The model under review builds one solid part; all positions refer to its coordinate system, in mm. Coordinates: 2 decimals unless noted, no trailing zeros. Order: outer loops, then holes, each group sorted by start corner. A loop starts at its lowest first (then second) coordinate and runs counter-clockwise, first axis right, second up. Notation, with made-up numbers: (-11.5, 41.5) -> (23.5, 41.5) arc R17 ccw to (23.5, 56.5) -> close; hole circle Ø6 at (82.25, 17). An arc over 180 degrees is marked (long way). Put each result on its own line as item: value.
from build123d import *

# Parameters (mm, degrees)
ESQUISSE1_R             = 32.5
BOSS_EXTRU_2_DEPTH      = 5
ESQUISSE2_R             = 2
ENL_V_MAT_EXTRU_1_DEPTH = 5
ENL_V_MAT_EXTRU_2_DEPTH = 10


with BuildPart() as part:
    # Esquisse1 → Boss.-Extru.2 (new body)
    with BuildSketch(Plane.XY):
        with BuildLine():
            Line((-2, 166.988023523), (-2, 99.979998))
            ThreePointArc((-2, 99.979998), (100, 0), (-2, -99.979998))
            Line((-2, -99.979998), (-2, -166.988023523))
            ThreePointArc((-2, -166.988023523), (167, 0), (-2, 166.988023523))
        make_face()
        with Locations((33.922197974, 129.118296475)):
            Circle(ESQUISSE1_R, mode=Mode.SUBTRACT)
        with Locations((93.936633435, 94.858625854)):
            Circle(ESQUISSE1_R, mode=Mode.SUBTRACT)
        with Locations((128.780823828, 35.18166304)):
            Circle(ESQUISSE1_R, mode=Mode.SUBTRACT)
        with Locations((129.118296475, -33.922197974)):
            Circle(ESQUISSE1_R, mode=Mode.SUBTRACT)
        with Locations((94.858625854, -93.936633435)):
            Circle(ESQUISSE1_R, mode=Mode.SUBTRACT)
        with Locations((35.18166304, -128.780823828)):
            Circle(ESQUISSE1_R, mode=Mode.SUBTRACT)
    extrude(amount=BOSS_EXTRU_2_DEPTH)

    # Esquisse2 → Enlèv. mat.-Extru.1 (cut)
    with BuildSketch(Plane(origin=(0, 0, 0), x_dir=(-1, 0, 0), z_dir=(0, 0, -1))):
        with Locations((-77.031940381, 134.503086066)):
            Circle(ESQUISSE2_R)
        with Locations((-54.667828657, 95.453803014)):
            Circle(ESQUISSE2_R)
        with Locations((-77.96711923, -133.963160305)):
            Circle(ESQUISSE2_R)
        with Locations((-55.33150397, -95.070629894)):
            Circle(ESQUISSE2_R)
        with Locations((-134.503086066, -77.031940381)):
            Circle(ESQUISSE2_R)
        with Locations((-95.453803014, -54.667828657)):
            Circle(ESQUISSE2_R)
        with Locations((-154.999059611, 0.53992576)):
            Circle(ESQUISSE2_R)
        with Locations((-109.999332627, 0.38317312)):
            Circle(ESQUISSE2_R)
        with Locations((-133.963160305, 77.96711923)):
            Circle(ESQUISSE2_R)
        with Locations((-95.070629894, 55.33150397)):
            Circle(ESQUISSE2_R)
    extrude(amount=-ENL_V_MAT_EXTRU_1_DEPTH, mode=Mode.SUBTRACT)

    # Esquisse3 → Enlèv. mat.-Extru.2 (cut)
    with BuildSketch(Plane.XY.offset(5)):
        Polygon((0, 0), (77.031940381, 134.503086066), (82.995703507, 144.916228213), (91.624548615, 157.474747761), (25.313830581, 172.484842021), (-36.151543954, 181.613524578), (-51.569744744, -183.237067308), (77.031940381, -179.146608877), (82.995703507, -170.83045621), (84.003283299, -144.334501748), (77.96711923, -133.963160305), align=None)
    extrude(amount=-ENL_V_MAT_EXTRU_2_DEPTH, mode=Mode.SUBTRACT)


solid = part.part
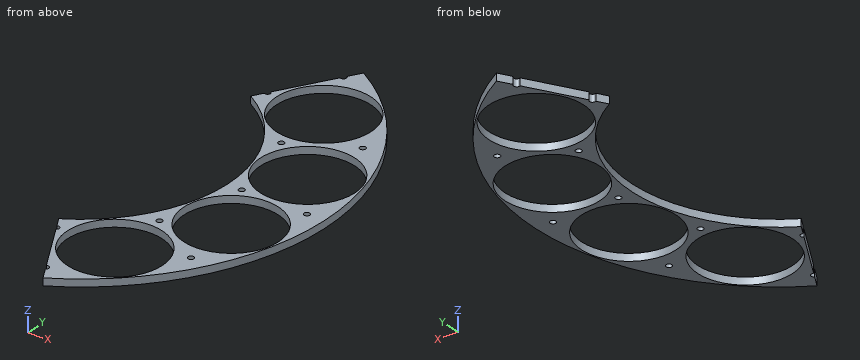
Item 1: For line 1 (Y direction, x = 129, z = 1.9); line 2 (Y direction, x = 129.5, z = 1.05); line 3 (Y direction, x = 83.5, z = 3.8) (3 decimals), list the stretches that pass through material, from the lowest coordinate up. Write a range as from..to.
Answers below:
line 1: -106.06..-66.42, -1.42..2.68, 67.68..106.06
line 2: -105.45..-66.42, -1.42..2.69, 67.67..105.45
line 3: -143.47..-124.387, -63.486..-55.025, 55.025..64.08, 125.637..144.626
Item 2: Consider section B-B on x = 105. Write out the cut boundary in (y, z).
Answers below:
outline: (-129.86, 0) -> (-124.81, 0) -> (-124.81, 5) -> (-129.86, 5) -> close; (-63.06, 0) -> (-55.71, 0) -> (-55.71, 5) -> (-63.06, 5) -> close; (-12.14, 0) -> (13.03, 0) -> (13.03, 5) -> (-12.14, 5) -> close; (57.33, 0) -> (64.3, 0) -> (64.3, 5) -> (57.33, 5) -> close; (125.42, 0) -> (129.86, 0) -> (129.86, 5) -> (125.42, 5) -> close
Item 3: Consider section A-A on y = 112.5. Write out the cut boundary in (x, z).
Answers below:
outline: (64.43, 0) -> (66.64, 0) -> (66.64, 5) -> (64.43, 5) -> close; (121.23, 0) -> (123.42, 0) -> (123.42, 5) -> (121.23, 5) -> close
Item 4: Consider section C-C on x = 70. Write out the cut boundary in (y, z).
Answers below:
outline: (-120.27, 0) -> (-114.87, 0) -> (-114.87, 5) -> (-120.27, 5) -> close; (-73, 0) -> (-71.41, 0) -> (-71.41, 5) -> (-73, 5) -> close; (71.41, 0) -> (72.87, 0) -> (72.87, 5) -> (71.41, 5) -> close; (116.84, 0) -> (122.22, 0) -> (122.22, 5) -> (116.84, 5) -> close
Item 5: Consider section D-D on z = 1. Count the separate pieces of the cut face and the enclosed holes in it, and give its area (3 significant figures).
Answers below:
separate pieces: 1
enclosed holes: 10
area: 5,360 mm^2
Item 6: For pin 1 Ø1.5 at (y, z) = (81.5, 3) entering from +X; pin 2 Ø2 at (x, z) = (138.5, 3.5) entering from +Y, all flat-tipped, find the tip position at first contact; note any pin that passes through.
Answers below:
pin 1: x = 146.18
pin 2: y = 94.78
